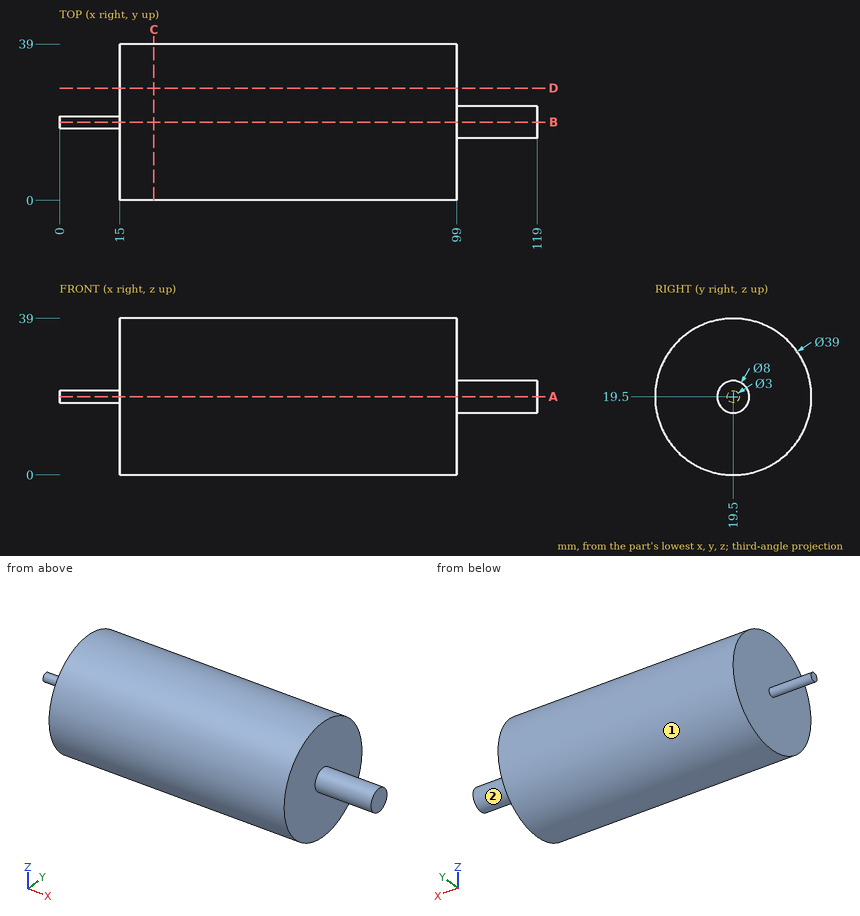
Design review of the part shown in the three views and the two pictorial views. Dimensions are in mm from the part's minimum x, y and z. A direction names the side the tool comes from. Round coordinates to 2 decimals unless told otherwise and drop trailing zeros. Order: outer loops, then holes, each group sorted by start corner. A loop starts at its lowest first (then second) coordinate and runs counter-clockwise, first axis right, second up.
Q1. We need section C-C, the plane x = 23.5. Give the boundary of the cut face in (y, z).
Findings below:
outline: circle Ø39 at (19.5, 19.5)
Q2. Insertion check: P1, Ø1.5, axis at x = 27, z = 27, coming from the -Y side; P2, Ø6, axis at x = 35, y = 33, coming from the +Z side; P3, Ø4, axis at y = 17.5, z = 12.5, coming from the +X side. Each pin has a flat end and moves straight along its axis. Give the tip position at first contact, or say it passes through.
Findings below:
P1: stops at y = 1.21
P2: stops at z = 35.93
P3: stops at x = 99
Q3. We need section A-A, the plane z = 19.5. Give the boundary of the cut face in (x, y), plus the area to 3 significant figures.
Findings below:
outline: (0, 18) - (15, 18) - (15, 0) - (99, 0) - (99, 15.5) - (119, 15.5) - (119, 23.5) - (99, 23.5) - (99, 39) - (15, 39) - (15, 21) - (0, 21) - close
area: 3,480 mm2
Q4. We need section D-D, the plane y = 28. Give the boundary of the cut face in (x, z), plus the area to 3 significant figures.
Findings below:
outline: (15, 1.95) - (99, 1.95) - (99, 37.05) - (15, 37.05) - close
area: 2,950 mm2
Q5. Machinability: for the marked faces 1 and 2, which of the approach directions +Z, -Z, +X, -X, +Y, -Y give a long, thin tool a straight path to every point of the face, cutting with its end or side? Answer none if there is none.
Findings below:
face 1: +X, -X
face 2: +X
Q6. Wall thickness on line 1 (X direction, y = 4.5, z = 11); line 2 (Z direction, x = 98, y = 24.5); line 3 (Y direction, x = 75, z = 34.5): over which ranges is each line inside the solid? List them lowest first.
Findings below:
line 1: x = 15 to 99
line 2: z = 0.65 to 38.35
line 3: y = 7.04 to 31.96
